from build123d import *

# Parameters (mm, degrees)
SKETCH1_W           = 138
SKETCH1_H           = 69
BOSS_EXTRUDE1_DEPTH = 4
FILLET1_R           = 34.5


with BuildPart() as part:
    # Sketch1 → Boss-Extrude1 (new body)
    with BuildSketch(Plane(origin=(0, 0, 0), x_dir=(1, 0, 0), z_dir=(0, 1, 0))):
        Rectangle(SKETCH1_W, SKETCH1_H)
    extrude(amount=BOSS_EXTRUDE1_DEPTH)

    # Fillet1
    fillet1_edges = [part.edges().sort_by_distance(p)[0] for p in [
        (69, 2, 34.5),
        (69, 2, -34.5),
        (-69, 2, -34.5),
        (-69, 2, 34.5),
    ]]
    fillet(fillet1_edges, radius=FILLET1_R - 0.0001)  # a hair under: the kernel refuses the full size


solid = part.part
CAD build for the part. Positions are in the model's coordinates, mm. Coordinates: 2 decimals unless noted, no trailing zeros. Order: outer loops, then holes, each group sorted by start corner. A loop starts at its lowest first (then second) coordinate and runs counter-clockwise, first axis right, second up.
Item 1: Band-saw the part on C-C on z = -26. List the corners of the cut face in (x, y), plus the area to 3 significant figures.
Check sheet entries:
outline: (-57.18, 0) - (57.18, 0) - (57.18, 4) - (-57.18, 4) - close
area: 457 mm2
Item 2: Pin check, flat tips, straight feed: pin 1 Ø2 at (y, z) = (3, -9.5) entering from -X; pin 2 Ø2 at (y, z) = (1.5, 2) entering from -X. Stop position of each tip, or through.
Check sheet entries:
pin 1: stops at x = -67.94
pin 2: stops at x = -68.99
Item 3: Drill centre lines: L1, parallel to X at y = 1.6, z = -1; L2, parallel to X at y = 1.3, z = 8.5; L3, parallel to Z at x = -36, y = 1.2. Where is each one in solid material? Low to high.
Check sheet entries:
L1: x = -68.99 to 68.99
L2: x = -67.94 to 67.94
L3: z = -34.47 to 34.47
Item 4: Band-saw the part on B-B on z = 14.5. List the corners of the cut face in (x, y), plus the area to 3 significant figures.
Check sheet entries:
outline: (-65.8, 0) - (65.8, 0) - (65.8, 4) - (-65.8, 4) - close
area: 526 mm2
